Design review of the part built by this model. Coordinates are the model's own, in mm. Face numbers are marked on the shaded views. A direction names the side the tool comes from. Round coordinates to 2 decimals unless told otherwise and drop trailing zeros. Order: outer loops, then holes, each group sorted by start corner. A loop starts at its lowest first (then second) coordinate and runs counter-clockwise, first axis right, second up. Notation, with made-up numbers: (24.25, 84) - (82.25, 84) arc R37 cw to (82.25, 122) - close; hole circle Ø5 at (68.5, 65). An arc over 180 degrees is marked (long way). Write item = value, one per line.
from build123d import *

# Parameters (mm, degrees)
SKETCH_1_W          = 26
SKETCH_1_H          = 24
SKETCH_1_R          = 1.959448434
EXTRUDE_1_DEPTH     = 26
SKETCH_2_W          = 24
SKETCH_2_H          = 24
CUT_EXTRUDE_1_DEPTH = 24
SKETCH_3_R          = 2.210837502
CUT_EXTRUDE_2_DEPTH = 24


with BuildPart() as part:
    # 草图1 → 凸台-拉伸1 (new body)
    with BuildSketch(Plane(origin=(0, 0, 0), x_dir=(1, 0, 0), z_dir=(0, 1, 0))):
        with Locations((0.263585178, -0.243309395)):
            Rectangle(SKETCH_1_W, SKETCH_1_H)
        with Locations(Location((9.763585178, -8.243309395, 0), (0, 0, 90))):
            Circle(SKETCH_1_R, mode=Mode.SUBTRACT)
        with Locations(Location((9.763585178, -0.243309395, 0), (0, 0, 90))):
            Circle(SKETCH_1_R, mode=Mode.SUBTRACT)
        with Locations(Location((9.763585178, 7.756690605, 0), (0, 0, 90))):
            Circle(SKETCH_1_R, mode=Mode.SUBTRACT)
        with Locations(Location((1.763585178, -8.243309395, 0), (0, 0, 90))):
            Circle(SKETCH_1_R, mode=Mode.SUBTRACT)
        with Locations(Location((1.763585178, -0.243309395, 0), (0, 0, 90))):
            Circle(SKETCH_1_R, mode=Mode.SUBTRACT)
        with Locations(Location((1.763585178, 7.756690605, 0), (0, 0, 90))):
            Circle(SKETCH_1_R, mode=Mode.SUBTRACT)
        with Locations(Location((-6.236414822, -8.243309395, 0), (0, 0, 90))):
            Circle(SKETCH_1_R, mode=Mode.SUBTRACT)
        with Locations(Location((-6.236414822, -0.243309395, 0), (0, 0, 90))):
            Circle(SKETCH_1_R, mode=Mode.SUBTRACT)
        with Locations(Location((-6.236414822, 7.756690605, 0), (0, 0, 90))):
            Circle(SKETCH_1_R, mode=Mode.SUBTRACT)
    extrude(amount=EXTRUDE_1_DEPTH)

    # 草图2 → 切除-拉伸1 (cut)
    with BuildSketch(Plane(origin=(0, 26, 0), x_dir=(1, 0, 0), z_dir=(0, 1, 0))):
        with Locations((1.263585178, -0.243309395)):
            Rectangle(SKETCH_2_W, SKETCH_2_H)
    extrude(amount=-CUT_EXTRUDE_1_DEPTH, mode=Mode.SUBTRACT)

    # 草图3 → 切除-拉伸2 (cut)
    with BuildSketch(Plane.ZY.offset(12.736414822)):
        with Locations((-7.756690605, 22.5)):
            Circle(SKETCH_3_R)
        with Locations((0.243309395, 22.5)):
            Circle(SKETCH_3_R)
        with Locations((8.243309395, 22.5)):
            Circle(SKETCH_3_R)
        with Locations((-7.756690605, 14.5)):
            Circle(SKETCH_3_R)
        with Locations((0.243309395, 14.5)):
            Circle(SKETCH_3_R)
        with Locations((8.243309395, 14.5)):
            Circle(SKETCH_3_R)
        with Locations((-7.756690605, 6.5)):
            Circle(SKETCH_3_R)
        with Locations((0.243309395, 6.5)):
            Circle(SKETCH_3_R)
        with Locations((8.243309395, 6.5)):
            Circle(SKETCH_3_R)
    extrude(amount=-CUT_EXTRUDE_2_DEPTH, mode=Mode.SUBTRACT)


solid = part.part
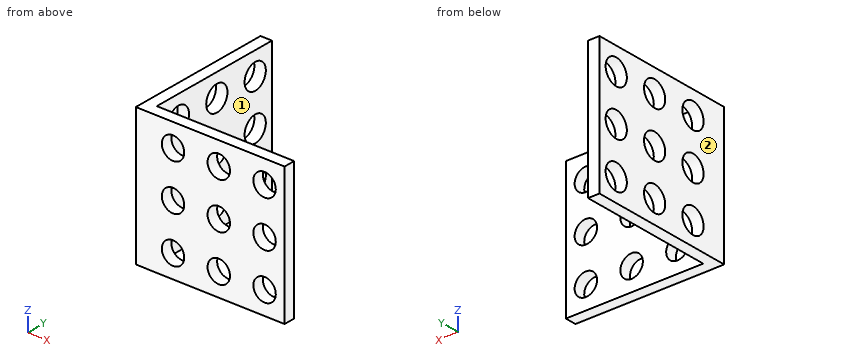
Item 1: Take a section at D-D, the plane z = 4.5. State the section outline as (x, y) points.
Data:
outline = (-12.74, 0) - (13.26, 0) - (13.26, 2) - (-10.74, 2) - (-10.74, 26) - (-12.74, 26) - close
Item 2: For line 1 along Y through (x, z) = (7.5, 5.5); line 2 along X through (y, z) = (12.5, -5.5), list the stretches that pass through material, from the lowest coordinate up. Write a range as [from, to].
Data:
line_1 = [0, 2]
line_2 = [-12.74, -10.74]
Item 3: Insertion check: P1, Ø5.5, axis at y = 14.5, z = 8.24, coming from the +X side; P2, Ø2.5, axis at y = 22.5, z = -7.76, coming from the -X side; P3, Ø2, axis at x = 9.5, z = -6, coming from the +Y side. Each pin has a flat end and moves straight along its axis. Give the tip position at first contact, or say it passes through.
Data:
P1 = -10.74
P2 = through
P3 = 2
Item 4: Take a section at A-A, the plane y = 22.5. State the section outline as (x, z) points.
Data:
outline = (-12.74, -11.76) - (-10.74, -11.76) - (-10.74, -9.97) - (-12.74, -9.97) - close; (-12.74, -5.55) - (-10.74, -5.55) - (-10.74, -1.97) - (-12.74, -1.97) - close; (-12.74, 2.45) - (-10.74, 2.45) - (-10.74, 6.03) - (-12.74, 6.03) - close; (-12.74, 10.45) - (-10.74, 10.45) - (-10.74, 12.24) - (-12.74, 12.24) - close
Item 5: Take a section at C-C, the plane z = -0.25. Count the separate pieces of the cut face and the enclosed holes in it, and give its area (3 significant figures).
Data:
separate_pieces = 7
enclosed_holes = 0
area = 51.4 mm2
Item 6: Take a section at B-B, the plane x = -7.75. State the section outline as (y, z) points.
Data:
outline = (0, -11.76) - (2, -11.76) - (2, -9) - (0, -9) - close; (0, -6.51) - (2, -6.51) - (2, -1) - (0, -1) - close; (0, 1.49) - (2, 1.49) - (2, 7) - (0, 7) - close; (0, 9.49) - (2, 9.49) - (2, 12.24) - (0, 12.24) - close
Item 7: For the marked faces 1 and 2, list the 3-axis set-ups (+Z, -Z, +X, -X, +Y, -Y) from which the entire face can be reached by the end or side of a thin tool; tool diameter is ignored.
Data:
face_1 = +Z, -Z, +X, +Y
face_2 = +Z, -Z, -X, +Y, -Y
